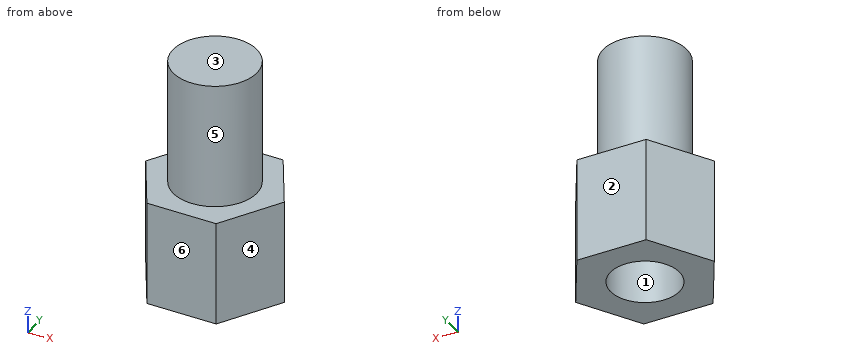
from build123d import *

# Parameters (mm, degrees)
EXTRUDE_1_DEPTH     = 5
SKETCH_2_R          = 2
EXTRUDE_2_DEPTH     = 6
SKETCH_3_R          = 1.65
CUT_EXTRUDE_1_DEPTH = 3


with BuildPart() as part:
    # 草圖1 → 填料-伸長1 (new body)
    with BuildSketch(Plane.XY):
        Polygon((-1.675, 2.901185103), (-3.35, 0), (-1.675, -2.901185103), (1.675, -2.901185103), (3.35, 0), (1.675, 2.901185103), align=None)
    extrude(amount=EXTRUDE_1_DEPTH)

    # 草圖2 → 填料-伸長2 (add)
    with BuildSketch(Plane.XY.offset(5)):
        Circle(SKETCH_2_R)
    extrude(amount=EXTRUDE_2_DEPTH)

    # 草圖3 → 除料-伸長1 (cut)
    with BuildSketch(Plane(origin=(0, 0, 0), x_dir=(-1, 0, 0), z_dir=(0, 0, -1))):
        Circle(SKETCH_3_R)
    extrude(amount=-CUT_EXTRUDE_1_DEPTH, mode=Mode.SUBTRACT)


solid = part.part
Input: part model. Units: mm. Frame: model coordinates. Face numbers are marked on the shaded views. A direction names the side the tool comes from. Round coordinates to 2 decimals unless told otherwise and drop trailing zeros. Write each loop counter-clockwise with the first axis right and the second up, starting at its lowest first coordinate (ties: lowest second). Pieces come first, ordered by that corner, then holes.
1) Cut plane B-B (y = -1). Return the cut outline in (x, z), then the cut area to 3 significant figures.
2) Ray query, L1, parallel to Y at x = 0, z = 0.75; L2, parallel to X at y = 0.2, z = 1; L3, parallel to Z at x = -0.25, y = 2.4. Return the intervals inside material, ascending.
3) Cut plane D-D (z = 6.5). Return the cut outline in (x, y), then the cut area to 3 significant figures.
4) Draft query along Y for the marked faces 1, 2, 3 and 4. Return one class per face: pulls with the +Y half, pulls with the -Y half, needs draft (parallel to the pull), parting line crosses it, or undercut.
5) Cut plane A-A (z = 4.25). Return the cut outline in (x, y) (3 decimals).
6) Reachability of the marked faces 5 and 6 from +Z, -Z, +X, -X, +Y, -Y: full face, straight path, thin tool, end or side. Return the list, or none.
7) Contact query for flat-ended pins moving along their axis: P1, Ø2.5, axis at x = -0.5, y = 1, coming from the -Z side; P2, Ø1, axis at y = -2, z = 3.5, coming from the -X side; P3, Ø1, axis at y = 0.5, z = 6, coming from the +X side. Output: stop coordinate, or through.
8) Cut plane C-C (x = 0). Return the cut outline in (y, z).
Geometry says:
1. outline: (-2.77, 0) - (-1.31, 0) - (-1.31, 3) - (1.31, 3) - (1.31, 0) - (2.77, 0) - (2.77, 5) - (1.73, 5) - (1.73, 11) - (-1.73, 11) - (-1.73, 5) - (-2.77, 5) - close
1. area: 40.6 mm2
2. L1: y = -2.9 to -1.65, 1.65 to 2.9
2. L2: x = -3.23 to -1.64, 1.64 to 3.23
2. L3: z = 0 to 5
3. outline: circle Ø4 at (0, 0)
3. area: 12.6 mm2
4. face 1: undercut
4. face 2: pulls with the +Y half
4. face 3: needs draft
4. face 4: pulls with the -Y half
5. outline: (-3.35, 0) - (-1.675, -2.901) - (1.675, -2.901) - (3.35, 0) - (1.675, 2.901) - (-1.675, 2.901) - close
6. face 5: +Z
6. face 6: +Z, -Z, +X, -X, -Y
7. P1: stops at z = 0
7. P2: stops at x = -2.48
7. P3: stops at x = 2
8. outline: (-2.9, 0) - (-1.65, 0) - (-1.65, 3) - (1.65, 3) - (1.65, 0) - (2.9, 0) - (2.9, 5) - (2, 5) - (2, 11) - (-2, 11) - (-2, 5) - (-2.9, 5) - close
